from build123d import *

# Parameters (mm, degrees)
SKETCH1_W           = 38
SKETCH1_H           = 10
SKETCH1_R           = 1.75
BOSS_EXTRUDE1_DEPTH = 12
CUT_EXTRUDE3_DEPTH  = 2


with BuildPart() as part:
    # Sketch1 → Boss-Extrude1 (new body)
    with BuildSketch(Plane.XY):
        Rectangle(SKETCH1_W, SKETCH1_H)
        with Locations((15, 1)):
            Circle(SKETCH1_R, mode=Mode.SUBTRACT)
        with Locations((-15, 1)):
            Circle(SKETCH1_R, mode=Mode.SUBTRACT)
    extrude(amount=BOSS_EXTRUDE1_DEPTH)

    # Sketch2 → Cut-Extrude3 (cut)
    with BuildSketch(Plane.XZ.offset(5)):
        with BuildLine():
            Line((2.2, -0.05), (2.2, 2.831644402))
            Line((2.2, 2.831644402), (14.549818203, 4.211125302))
            ThreePointArc((14.549818203, 4.211125302), (16.15, 6), (14.549818203, 7.788874698))
            Line((14.549818203, 7.788874698), (2.2, 9.168355598))
            Line((2.2, 9.168355598), (2.2, 12.75))
            ThreePointArc((2.2, 12.75), (0, 14.95), (-2.2, 12.75))
            Line((-2.2, 12.75), (-2.2, 9.713852446))
            Line((-2.2, 9.713852446), (-17.179844816, 7.785265067))
            ThreePointArc((-17.179844816, 7.785265067), (-18.75, 6), (-17.179844816, 4.214734933))
            Line((-17.179844816, 4.214734933), (-2.2, 2.286147554))
            Line((-2.2, 2.286147554), (-2.2, -0.05))
            ThreePointArc((-2.2, -0.05), (0, -2.25), (2.2, -0.05))
        make_face()
    extrude(amount=-CUT_EXTRUDE3_DEPTH, mode=Mode.SUBTRACT)


solid = part.part
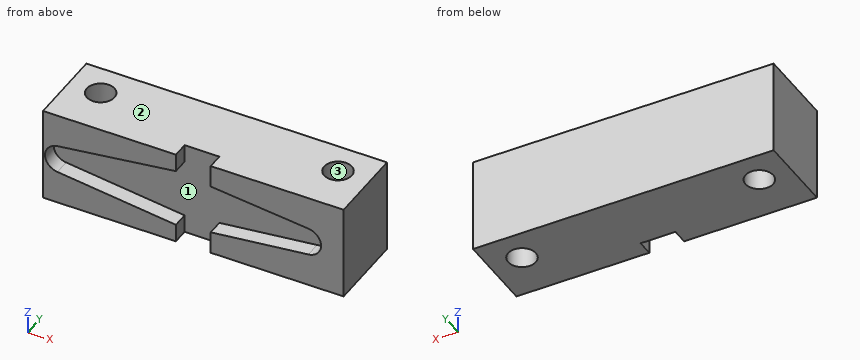
Could you check a few things on this model? Use its own coordinates, in mm. Face numbers are marked on the shaded views. Give positions to 0.01 mm unless a question says otherwise; leave off trailing zeros. Order: outer loops, then holes, each group sorted by start corner. A loop starts at its lowest first (then second) coordinate and runs counter-clockwise, first axis right, second up. Notation, with made-up numbers: (-27.5, 77.5) - (-22.5, 77.5) arc R6 cw to (-22.5, 81.5) - close; hole circle Ø5 at (74.5, -32). An arc over 180 degrees is marked (long way). One line per item, written item: value. Start each with the question number.
1. Imagine slicing it at B-B on y = 1. List the corners of the cut face in (x, z) for me.
2. Imagine slicing it at A-A on y = -4.5. List the corners of the cut face in (x, z) for me, plus the area to 3 significant figures.
3. Imagine slicing it at D-D on x = -15. List the corners of the cut face in (y, z) for me, plus the area to 3 significant figures.
4. Imagine slicing it at C-C on z = 10.5. List the corners of the cut face in (x, y) for me, plus the area to 3 significant figures.
5. Thinking about a two-plate mould opening in Y: for the marked faces 1, 2 and 3, which applies, +Y half, -Y half, draft (parallel to the pull), parting line (faces both ways), or undercut?
6. For P1, Ø4.5, axis at x = 15, y = 1, coming from the -Z side; P2, Ø1.5, axis at x = 1, z = 7, coming from the -Y side, each with a flat end and sliding along its axis, tell me the tip position at first contact or that it passes through.
7. If I drill on probe 1 along X at (y, z) = (-4.5, 10.25); probe 2 along Y at (x, z) = (-15, 5.5); probe 3 along X at (y, z) = (0.5, 2.5), over which ranges is the centre line in solid material (lowest first)?
Values:
1. outline: (-19, 0) - (-16.75, 0) - (-16.75, 12) - (-19, 12) - close; (-13.25, 0) - (13.25, 0) - (13.25, 12) - (-13.25, 12) - close; (16.75, 0) - (19, 0) - (19, 12) - (16.75, 12) - close
2. outline: (-19, 0) - (-2.2, 0) - (-2.2, 2.29) - (-17.18, 4.21) arc R1.8 cw to (-17.18, 7.79) - (-2.2, 9.71) - (-2.2, 12) - (-19, 12) - close; (2.2, 0) - (19, 0) - (19, 12) - (2.2, 12) - (2.2, 9.17) - (14.55, 7.79) arc R1.8 cw to (14.55, 4.21) - (2.2, 2.83) - close
2. area: 251 mm²
3. outline: (-5, 0) - (-0.75, 0) - (-0.75, 12) - (-5, 12) - (-5, 8.07) - (-3, 8.07) - (-3, 3.93) - (-5, 3.93) - close; (2.75, 0) - (5, 0) - (5, 12) - (2.75, 12) - close
3. area: 69.7 mm²
4. outline: (-19, -5) - (-2.2, -5) - (-2.2, -3) - (2.2, -3) - (2.2, -5) - (19, -5) - (19, 5) - (-19, 5) - close; hole circle Ø3.5 at (-15, 1); hole circle Ø3.5 at (15, 1)
4. area: 352 mm²
5. face 1: -Y half
5. face 2: draft
5. face 3: undercut
6. P1: z = 0
6. P2: y = -3
7. probe 1: -19 to -2.2, 2.2 to 19
7. probe 2: -3 to -0.75, 2.75 to 5
7. probe 3: -19 to -16.68, -13.32 to 13.32, 16.68 to 19
